```python
from build123d import *

# Parameters (mm, degrees)
SKETCH1_W           = 2.6797
SKETCH1_H           = 0.9906
SKETCH2_R           = 1.4478
BOSS_EXTRUDE1_DEPTH = 7.9375
CUT_EXTRUDE1_DEPTH  = 0.5588
CHAMFER1_SIZE       = 0.254
FILLET1_R           = 0.254
FILLET2_R           = 0.5588


with BuildPart() as part:
    # Sketch1 → Revolve1 (revolve)
    with BuildSketch(Plane.XY):
        with Locations((1.33985, 0.4953)):
            Rectangle(SKETCH1_W, SKETCH1_H)
    revolve(axis=Axis((0, 0.9906, 0), (0, -1, 0)))

    # Sketch2 → Boss-Extrude1 (add)
    with BuildSketch(Plane.XZ):
        Circle(SKETCH2_R)
    extrude(amount=BOSS_EXTRUDE1_DEPTH)

    # Sketch3 → Cut-Extrude1 (cut)
    with BuildSketch(Plane(origin=(0, 0.9906, 0), x_dir=(-1, 0, 0), z_dir=(0, 1, 0))):
        Polygon((-0.5715, -0.5715), (-0.5715, -1.905), (0.5715, -1.905), (0.5715, -0.5715), (1.905, -0.5715), (1.905, 0.5715), (0.5715, 0.5715), (0.5715, 1.905), (-0.5715, 1.905), (-0.5715, 0.5715), (-1.905, 0.5715), (-1.905, -0.5715), align=None)
    extrude(amount=-CUT_EXTRUDE1_DEPTH, mode=Mode.SUBTRACT)

    # Chamfer1
    chamfer1_edges = [part.edges().sort_by_distance(p)[0] for p in [
        (-1.4478, -7.9375, 0),
    ]]
    chamfer(chamfer1_edges, length=CHAMFER1_SIZE)

    # Fillet1
    fillet1_edges = [part.edges().sort_by_distance(p)[0] for p in [
        (-1.4478, 0, 0),
    ]]
    fillet(fillet1_edges, radius=FILLET1_R)

    # Fillet2
    fillet2_edges = [part.edges().sort_by_distance(p)[0] for p in [
        (-2.6797, 0.9906, 0),
    ]]
    fillet(fillet2_edges, radius=FILLET2_R)


solid = part.part
```
Design review of the part built by this model. Coordinates are the model's own, in mm. A direction names the side the tool comes from. Round coordinates to 2 decimals unless told otherwise and drop trailing zeros. Order: outer loops, then holes, each group sorted by start corner. A loop starts at its lowest first (then second) coordinate and runs counter-clockwise, first axis right, second up. Notation, with made-up numbers: (89.25, 59.5) - (104.25, 59.5) arc R27 ccw to (104.25, 84.5) - close; hole circle Ø7 at (15, 69). An arc over 180 degrees is marked (long way). Return JSON: item names as keys, results as strings.
Q1. Wall thickness on L1, parallel to X at y = 0.75, z = 1.35; L2, parallel to X at y = -3.5, z = -0.05; L3, parallel to X at y = 0.5, z = 0.1 (3 decimals): over which ranges is each line inside the solid? List them lowest first. Write a range as [from, to].
Computed values:
{"L1": "x = [-2.2, -0.57], [0.57, 2.2]", "L2": "x = [-1.45, 1.45]", "L3": "x = [-2.674, -1.905], [1.905, 2.674]"}
Q2. Machinability: for faces 4 (the flat face through (0, 0, -2)), 5 (the cylindrical face through (-2.677, 0.219, 0.118)), which of the approach directions +Z, -Z, +X, -X, +Y, -Y give a long, thin tool a straight path to every point of the face, cutting with its end or side? Answer none if there is none.
Computed values:
{"face 4": "-Y", "face 5": "+Y, -Y"}
Q3. The part is to be moulded in two halves that separate along X. For faces 1 (the flat face through (-1, 0.991, -1)), 2 (the flat face through (0, 0.432, 0)), 3 (the cylindrical face through (-0.314, -3.917, -1.413)), say which applies: pulls with the +X half, pulls with the -X half, needs draft (parallel to the pull), parting line crosses it, or undercut.
Computed values:
{"face 1": "needs draft", "face 2": "undercut", "face 3": "parting line crosses it"}
Q4. For pin 1 Ø1 at (y, z) = (-1, 0) entering from -X; pin 2 Ø0.6 at (y, z) = (1, 0) entering from +X; pin 3 Ø2 at (y, z) = (-2.5, -1.5) entering from +X, all flat-tipped, find the tip position at first contact; note any pin that passes through.
Computed values:
{"pin 1": "stops at x = -1.45", "pin 2": "stops at x = 2.61", "pin 3": "stops at x = 1.36"}
Q5. Consider section C-C on y = -5.25. Write out the cut boundary in (x, z).
Computed values:
{"outline": "circle Ø2.9 at (0, 0)"}
